For this review, take the finished solid that the model builds, in its own axes (mm). Coordinates: 2 decimals unless noted, no trailing zeros. Loops run counter-clockwise (first coordinate to the right, second up) from the corner with the lowest first, then second, coordinate; pieces in that order, holes last. Notation, with made-up numbers: (-19.75, -32) -> (21.25, -32) arc R5 ccw to (21.25, -24) -> close; hole circle Ø3 at (3, 50). An arc over 180 degrees is marked (long way). Answer in a Markdown table with one row per item.
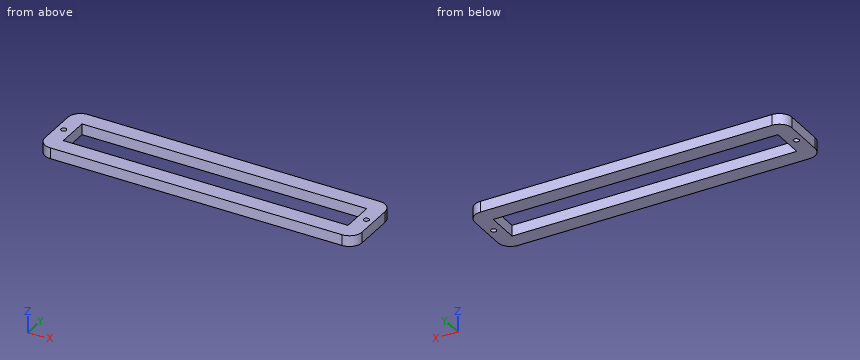
Autodesk Fusion 360 part; units mm, degrees
sketch "Sketch1" plane through (0, 0, 0) normal (0, 0, 1) x (1, 0, 0)
  line L0 (-79, 9) -> (79, 9)
  line L1 (79, 9) -> (79, -9)
  line L2 (79, -9) -> (-79, -9)
  line L3 (-79, -9) -> (-79, 9)
  line L4 (-79, 9) -> (79, -9) construction
  line L5 (79, 9) -> (-79, -9) construction
  line L6 (-81, 18) -> (81, 18)
  line L7 (88, 11) -> (88, -11)
  line L8 (81, -18) -> (-81, -18)
  line L9 (-88, -11) -> (-88, 11)
  line L10 (-88, 18) -> (88, -18) construction
  line L11 (88, 18) -> (-88, -18) construction
  arc A0 (-81, 18) -> (-88, 11) centre (-81, 11) ccw
  arc A1 (-88, -11) -> (-81, -18) centre (-81, -11) ccw
  arc A2 (81, -18) -> (88, -11) centre (81, -11) ccw
  arc A3 (88, 11) -> (81, 18) centre (81, 11) ccw
  line L12 (0, 0) -> (27, 0) construction
  circle A4 centre (-84, 0) radius 1.5
  line L13 (0, 0) -> (0, 18) construction
  circle A5 centre (84, 0) radius 1.5
  dimension "d22" = 158
  dimension "d23" = 18
  dimension "d28" = 176
  dimension "d29" = 36
  dimension "d30" = 7
  dimension "d35" = 3
  dimension "d37" = 18
  dimension "d54" = 5
extrude "Extrude7" add sketch "Sketch1" along normal blind 6
sketch "Sketch3" plane through (0, 0, 3) normal (0, 0, 1) x (-1, 0, 0)
  circle A0 centre (0, -13) radius 1.5
  circle A1 centre (-85, 0) radius 1.5
  circle A2 centre (0, 13) radius 1.5
  circle A3 centre (85, 0) radius 1.5
  line L0 (-79, 9) -> (79, 9)
  line L1 (79, 9) -> (79, -9)
  line L2 (79, -9) -> (-79, -9)
  line L3 (-79, -9) -> (-79, 9)
  arc A4 (-83, 18) -> (-90, 11) centre (-83, 11) ccw
  line L4 (-90, 11) -> (-90, -11)
  arc A5 (-90, -11) -> (-83, -18) centre (-83, -11) ccw
  line L5 (-83, -18) -> (83, -18)
  arc A6 (83, -18) -> (90, -11) centre (83, -11) ccw
  line L6 (90, -11) -> (90, 11)
  arc A7 (90, 11) -> (83, 18) centre (83, 11) ccw
  line L7 (83, 18) -> (-83, 18)
  circle A8 centre (0, 13) radius 1.5
Item 1: Take a section at C-C, the plane z = 3.3. State the section outline as (x, y) points.
Worked answers:
| item | result |
|---|---|
| outline | (-88, -11) arc R7 ccw to (-81, -18) -> (81, -18) arc R7 ccw to (88, -11) -> (88, 11) arc R7 ccw to (81, 18) -> (-81, 18) arc R7 ccw to (-88, 11) -> close; hole circle Ø3 at (-84, 0); hole (-79, -9) -> (79, -9) -> (79, 9) -> (-79, 9) -> close; hole circle Ø3 at (84, 0) |
Item 2: Take a section at A-A, the plane y = 0. State the section outline as (x, z) points, and give its area (3 significant figures).
Worked answers:
| item | result |
|---|---|
| outline | (-88, 0) -> (-85.5, 0) -> (-85.5, 6) -> (-88, 6) -> close; (-82.5, 0) -> (-79, 0) -> (-79, 6) -> (-82.5, 6) -> close; (79, 0) -> (82.5, 0) -> (82.5, 6) -> (79, 6) -> close; (85.5, 0) -> (88, 0) -> (88, 6) -> (85.5, 6) -> close |
| area | 72.0 mm² |
Item 3: Take a section at D-D, the plane x = -84. State the section outline as (y, z) points.
Worked answers:
| item | result |
|---|---|
| outline | (-17.32, 0) -> (-1.5, 0) -> (-1.5, 6) -> (-17.32, 6) -> close; (1.5, 0) -> (17.32, 0) -> (17.32, 6) -> (1.5, 6) -> close |
Item 4: For L1, parallel to Y at x = 72, z = 5.4; L2, parallel to X at y = -8.5, z = 2.95; L3, parallel to Y at x = -84, z = 4, list the stretches that pass through material, from the lowest coordinate up.
Worked answers:
| item | result |
|---|---|
| L1 | -18 to -9, 9 to 18 |
| L2 | -88 to -79, 79 to 88 |
| L3 | -17.32 to -1.5, 1.5 to 17.32 |
Item 5: Take a section at B-B, the plane x = 4.5. State the section outline as (y, z) points, and give its area (3 significant figures).
Worked answers:
| item | result |
|---|---|
| outline | (-18, 0) -> (-9, 0) -> (-9, 6) -> (-18, 6) -> close; (9, 0) -> (18, 0) -> (18, 6) -> (9, 6) -> close |
| area | 108 mm² |
